```python
from build123d import *

# Parameters (mm, degrees)
SKETCH001_R     = 2
PAD_DEPTH       = 5
SKETCH_W        = 13.5
SKETCH_H        = 4
PAD001_DEPTH    = 24
SKETCH002_W     = 13.5
SKETCH002_H     = 4
PAD002_DEPTH    = 10
SKETCH003_R     = 1.5
POCKET_DEPTH    = 5
CHAMFER_SIZE    = 1.5
CHAMFER001_SIZE = 2.5
FILLET_R        = 16


with BuildPart() as part:
    # Sketch001 → Pad (new body)
    with BuildSketch(Plane.XZ):
        with BuildLine():
            Line((-22.5, 33), (22.5, 33))
            Line((22.5, 33), (22.5, 0))
            Line((9, 0), (22.5, 0))
            Line((9, 6.503914), (9, 0))
            ThreePointArc((9, 6.503914), (0, 32.6), (-9, 6.503914))
            Line((-9, 0), (-9, 6.503914))
            Line((-22.5, 0), (-9, 0))
            Line((-22.5, 0), (-22.5, 33))
        make_face()
        with Locations((-17.5, 18)):
            Circle(SKETCH001_R, mode=Mode.SUBTRACT)
        with Locations((17.5, 18)):
            Circle(SKETCH001_R, mode=Mode.SUBTRACT)
    extrude(amount=PAD_DEPTH)

    # Sketch (on Face12 of Pad) → Pad001 (join)
    with BuildSketch(Plane.XZ.offset(5)):
        with Locations((-15.75, 2)):
            Rectangle(SKETCH_W, SKETCH_H)
        with Locations((15.75, 2)):
            Rectangle(SKETCH_W, SKETCH_H)
    extrude(amount=PAD001_DEPTH)

    # Sketch002 (on Face1 of Pad001) → Pad002 (join)
    with BuildSketch(Plane(origin=(0, 0, 0), x_dir=(1, 0, 0), z_dir=(0, 1, 0))):
        with Locations((-15.75, -2)):
            Rectangle(SKETCH002_W, SKETCH002_H)
        with Locations((15.75, -2)):
            Rectangle(SKETCH002_W, SKETCH002_H)
    extrude(amount=PAD002_DEPTH)

    # Sketch003 (on Face6 of Pad002) → Pocket (cut)
    with BuildSketch(Plane(origin=(0, 0, 4), x_dir=(-1, 0, 0), z_dir=(0, 0, 1))):
        with Locations((-16, 19)):
            Circle(SKETCH003_R)
        with Locations((16, 19)):
            Circle(SKETCH003_R)
        with Locations((-16, -6)):
            Circle(SKETCH003_R)
        with Locations((16, -6)):
            Circle(SKETCH003_R)
    extrude(amount=-POCKET_DEPTH, mode=Mode.SUBTRACT)

    # Chamfer
    chamfer_edges = [part.edges().sort_by_distance(p)[0] for p in [
        (-14.5, -19, 4),
        (17.5, -19, 4),
        (-14.5, 6, 4),
        (17.5, 6, 4),
    ]]
    chamfer(chamfer_edges, length=CHAMFER_SIZE)

    # Chamfer001
    chamfer001_edges = [part.edges().sort_by_distance(p)[0] for p in [
        (-15.75, -5, 4),
        (15.75, -5, 4),
        (15.75, 0, 4),
        (-15.75, 0, 4),
    ]]
    chamfer(chamfer001_edges, length=CHAMFER001_SIZE)

    # Fillet
    fillet_edges = [part.edges().sort_by_distance(p)[0] for p in [
        (-22.5, -2.5, 33),
        (22.5, -2.5, 33),
    ]]
    fillet(fillet_edges, radius=FILLET_R)


solid = part.part
```
For this review, take the finished solid that the model builds, in its own axes (mm). A direction names the side the tool comes from. Round coordinates to 2 decimals unless told otherwise and drop trailing zeros. Write each loop counter-clockwise with the first axis right and the second up, starting at its lowest first coordinate (ties: lowest second). Pieces come first, ordered by that corner, then holes.
1) Take a section at A-A on y = -8.5. Give the boundary of the cut face in (x, z), then the cut area to 3 significant figures.
Answer below:
outline: (-22.5, 0) - (-9, 0) - (-9, 4) - (-22.5, 4) - close; (9, 0) - (22.5, 0) - (22.5, 4) - (9, 4) - close
area: 108 mm2
2) Insertion check: pin 1 Ø13 at (x, z) = (-6, 23.5) entering from +Y; pin 2 Ø5 at (x, z) = (17, 18.5) entering from -Y; pin 3 Ø4 at (x, y) = (18, -14) entering from +Z; pin 4 Ø1.5 at (y, z) = (2.5, 21) entering from +X. Each pin has a flat end and moves straight along its axis. Give the tip position at first contact, or say it passes through.
Answer below:
pin 1: stops at y = 0
pin 2: stops at y = -5
pin 3: stops at z = 4
pin 4: passes through
3) Mouldability with a two-part tool opening along X and no side actions: class faces 1 (the face through (-22.5, -7, 4)), 2 (the face through (-14, 6, 3)), 3 (the face through (16, 10, 2)), 4 (the face through (22.5, -5, 5)) as +X half, -X half, draft (parallel to the pull), parting line (faces both ways), or undercut.
Answer below:
face 1: -X half
face 2: undercut
face 3: draft
face 4: +X half
4) Take a section at D-D on y = -4. Give the boundary of the cut face in (x, z), then the cut area to 3 significant figures.
Answer below:
outline: (-22.5, 0) - (-9, 0) - (-9, 6.5) arc R14.6 cw (long way) to (9, 6.5) - (9, 0) - (22.5, 0) - (22.5, 17) arc R16 ccw to (6.5, 33) - (-6.5, 33) arc R16 ccw to (-22.5, 17) - close; hole circle Ø4 at (-17.5, 18); hole circle Ø4 at (17.5, 18)
area: 601 mm2
5) For line 1 along X through (y, z) = (6, 1); line 2 along Y through (x, z) = (-16, 1); line 3 along Z through (x, y) = (-11, -9), list the stretches that pass through material, from the lowest coordinate up.
Answer below:
line 1: x = -22.5 to -17.5, -14.5 to -9, 9 to 14.5, 17.5 to 22.5
line 2: y = -29 to -20.5, -17.5 to 4.5, 7.5 to 10
line 3: z = 0 to 4
6) Take a section at C-C on y = -19. Give the boundary of the cut face in (x, z), then the cut area to 3 significant figures.
Answer below:
outline: (-22.5, 0) - (-17.5, 0) - (-17.5, 2.5) - (-19, 4) - (-22.5, 4) - close; (-14.5, 0) - (-9, 0) - (-9, 4) - (-13, 4) - (-14.5, 2.5) - close; (9, 0) - (14.5, 0) - (14.5, 2.5) - (13, 4) - (9, 4) - close; (17.5, 0) - (22.5, 0) - (22.5, 4) - (19, 4) - (17.5, 2.5) - close
area: 79.5 mm2
7) Machinability: for faces 5 (the face through (-14.5, 5.93, 1.27)), 6 (the face through (9, -9, 3)), 7 (the face through (15.7, -15.7, 4)), 8 (the face through (-14, 9, 4)), 9 (the face through (0.51, -2.46, 32.59)), which of the approach directions +Z, -Z, +X, -X, +Y, -Y give a long, thin tool a straight path to every point of the face, cutting with its end or side? Answer none if there is none.
Answer below:
face 5: +Z, -Z
face 6: -Z, +Y, -Y
face 7: +Z, +X, -X, -Y
face 8: +Z, +X, -X, +Y
face 9: +Y, -Y
8) Take a section at B-B on z = 9.5. Give the boundary of the cut face in (x, y), then the cut area to 3 significant figures.
Answer below:
outline: (-22.5, -5) - (-11.87, -5) - (-11.87, 0) - (-22.5, 0) - close; (11.87, -5) - (22.5, -5) - (22.5, 0) - (11.87, 0) - close
area: 106 mm2
